Build history of the part. All positions in model axes, mm. Round coordinates to 2 decimals unless told otherwise and drop trailing zeros. Order: outer loops, then holes, each group sorted by start corner. A loop starts at its lowest first (then second) coordinate and runs counter-clockwise, first axis right, second up. Notation, with made-up numbers: (7, -30) -> (40, -30) arc R19 cw to (40, -11) -> close; hole circle Ø2 at (46.25, 24.5). An arc over 180 degrees is marked (long way). Use a Markdown table: item, result. Add a question column.
Item 1: Slice it at A-A, the plane z = 39.5. Give the cut face in (x, y).
Item 2: Pin check, flat tips, straight feed: pin 1 (2 mm diameter, centred on x = 3, z = 62, fed in from +Y); pin 2 (2.5 mm diameter, centred on y = 2, z = 70.5, fed in from -X); pin 3 (1 mm diameter, centred on x = -4, y = 4.5, fed in from +Z); pin 4 (1.6 mm diameter, centred on y = 2, z = 49.5, fed in from +X). Stop position of each tip, or through.
Item 3: Slice it at C-C, the plane z = -32. Give the cut face in (x, y), plus the area to 3 significant figures.
Item 4: Slice it at D-D, the plane y = 4.25. State how many separate pieces and enclosed holes the cut face has, plus the area to 3 significant figures.
Item 5: Probe L1, parallel to X at y = 4.55, z = 72; L2, parallel to X at y = 1.5, z = 43.5; L3, parallel to X at y = 3.25, z = 11.5. List the from-to ranges inside material, lowest first.
Item 6: Slice it at B-B, the plane x = 0. Give the cut face in (y, z), plus the area to 3 significant figures.
Autodesk Inventor part; units mm, degrees
ref_plane "YZ Plane" through (0, 0, 0) normal (1, 0, 0) x (0, 1, 0)
ref_plane "XZ Plane" through (0, 0, 0) normal (0, 1, 0) x (-1, 0, 0)
ref_plane "XY Plane" through (0, 0, 0) normal (0, 0, 1) x (1, 0, 0)
sketch "Boceto1" plane through (0, 0, 0) normal (0, 1, 0) x (-1, 0, 0)
  line L0 (26.7996, 74.6) -> (26.8, 68.8)
  line L1 (21, 68.8) -> (21, 22.2711)
  line L2 (7.5058, -28.0118) -> (9.0069, -33.6142)
  line L3 (-9.0069, -33.6142) -> (-7.5058, -28.0118)
  line L4 (-7.5058, -28.0118) -> (-9.0069, -33.6142)
  line L5 (-20.5061, -20.5061) -> (-24.6073, -24.6073)
  line L6 (-20.5061, -20.5061) -> (-24.6073, -24.6073)
  circle A0 centre (0, 0) radius 11
  line L7 (-21, 69) -> (-21, 22.2711)
  line L8 (-21, 22.2711) -> (-21, 69)
  line L9 (-26.7402, 22.2711) -> (-21, 22.2711)
  line L10 (-27, 74.8) -> (26.7996, 74.6)
  arc A1 (-9.0069, -33.6142) -> (9.0069, -33.6142) centre (0, 0) ccw
  arc A2 (-26.7402, 22.2711) -> (-24.6073, -24.6073) centre (0, 0) ccw
  arc A3 (24.6073, -24.6073) -> (26.7402, 22.2711) centre (0, 0) ccw
  line L11 (26.8, 68.8) -> (21, 68.8)
  line L12 (21, 22.2711) -> (26.7402, 22.2711)
  line L13 (-27, 74.8) -> (-27, 69)
  line L14 (-27, 69) -> (-21, 69)
  line L15 (24.6073, -24.6073) -> (20.3647, -20.3647)
  line L16 (7.5058, -28.0118) -> (7.454, -27.8187)
  line L17 (-7.5058, -28.0118) -> (-7.454, -27.8187)
  line L18 (-20.5061, -20.5061) -> (-20.3647, -20.3647)
  arc A4 (-20.3647, -20.3647) -> (-7.454, -27.8187) centre (0, 0) ccw
  arc A5 (7.454, -27.8187) -> (20.3647, -20.3647) centre (0, 0) ccw
  point P0 (0, 0)
  point P1 (0, 0)
  dimension "d3" = 53.8
  dimension "d5" = 22
  dimension "d15" = 5.8
  dimension "d16" = 46.5289
extrude "Extrusión1" add sketch "Boceto1" along normal blind 6
fillet "Empalme2" radius 1 2 edges at (27, 3, 74.8) (-26.7996, 3, 74.6)
chamfer "Chaflán1" distance 0.6 angle 45 6 edges at (27, 0, 71.3981) (26.7058, 0, 74.5047) (0.0964, 0, 74.7) (-26.5081, 0, 74.3095) (-26.7998, 0, 71.2019) (24, 0, 69)
chamfer "Chaflán2" distance 0.6 angle 45 1 edges at (21, 0, 45.6355)
chamfer "Chaflán3" distance 0.6 angle 45 1 edges at (-21, 0, 45.5355)
chamfer "Chaflán4" distance 0.6 angle 45 2 edges at (-23.6, 0, 68.8) (-23.8701, 0, 22.2711)
chamfer "Chaflán5" distance 0.6 angle 45 3 edges at (-34.7443, 0, -1.9681) (-24.1144, 0, 21.6711) (-22.486, 0, -22.486)
chamfer "Chaflán6" distance 0.6 angle 45 9 edges at (-14.4, 0, -24.9415) (-8.2563, 0, -30.813) (0, 0, -34.8) (8.2563, 0, -30.813) (14.4, 0, -24.9415) (22.5567, 0, -22.5567) (34.764, 0, -1.5817) (23.8701, 0, 22.2711) (20.4, 0, 45.6355)
fillet "Empalme4" radius 0.5 4 edges at (-9.0069, 3.2998, -33.6142) (-24.6073, 3.2998, -24.6073) (9.0069, 3.2998, -33.6142) (24.6073, 3.2998, -24.6073)
sketch "Boceto2" plane through (0, 0, 0) normal (0, -1, 0) x (1, 0, 0)
  line L0 (0, 52.5) -> (0, 37.5) construction
  line L1 (-12.5, 52.5) -> (-12.5, 37.5)
  line L2 (12.5, 37.5) -> (12.5, 52.5)
  arc A0 (12.5, 52.5) -> (-12.5, 52.5) centre (0, 52.5) ccw
  arc A1 (-12.5, 37.5) -> (12.5, 37.5) centre (0, 37.5) ccw
  point P0 (0, 0)
  point P1 (0, 45)
  dimension "d43" = 25
  dimension "d44" = 15
  dimension "d45" = 37.5
extrude "Extrusión2" cut sketch "Boceto2" against normal blind 6
sketch "Boceto3" plane through (0, 6, 0) normal (0, 1, 0) x (1, 0, 0)
  circle A0 centre (0.0066, -72) radius 1.6
  circle A1 centre (0, 0) radius 32
  circle A2 centre (0, 32) radius 1.6
  circle A3 centre (-30.0702, -10.9446) radius 1.6
  circle A4 centre (30.0702, -10.9446) radius 1.6
  line L0 (0, 0) -> (-30.0702, -10.9446)
  line L1 (0, 0) -> (30.0702, -10.9446)
  line L2 (9.4586, 0) -> (-7.7353, 0)
  dimension "d48" = 64
  dimension "d49" = 3.2
  dimension "d50" = 20
  dimension "d51" = 20
  dimension "d53" = 72
extrude "Extrusión3" cut sketch "Boceto3" against normal through all contours A0 | A2 A1 | A1 A2 | A4 A1 | A1 L1 A4 | A1 A4 L1 | A3 L0 A1 | A1 A3 | L0 A3 A1
properties part number "Tapa de caja reductora - eje z" material "Plastico PETG"
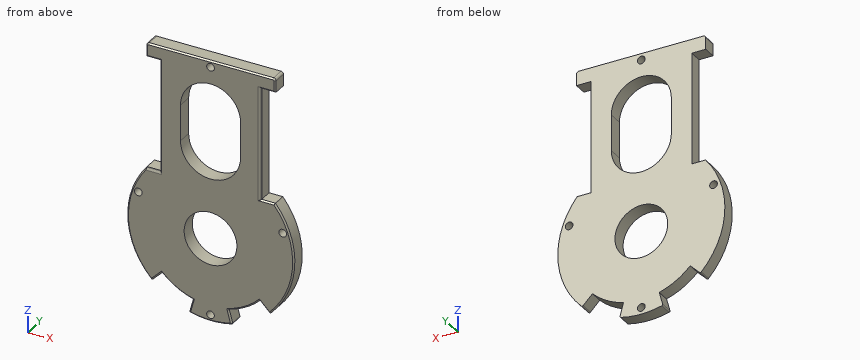
Check sheet entries:
| question | item | result |
|---|---|---|
| 1 | outline | (-21, 0.6) -> (-20.4, 0) -> (-12.5, 0) -> (-12.5, 6) -> (-21, 6) -> close; (12.5, 0) -> (19.8, 0) -> (20.82, 0.42) -> (21, 0.6) -> (21, 6) -> (12.5, 6) -> close |
| 2 | pin 1 | through |
| 2 | pin 2 | x = -26.8 |
| 2 | pin 3 | z = 74.69 |
| 2 | pin 4 | x = 21 |
| 3 | outline | (-8.57, 0.6) -> (-7.96, 0) -> (-1.6, 0) -> (-1.6, 6) -> (-8.57, 6) -> close; (1.6, 0) -> (7.96, 0) -> (8.57, 0.6) -> (8.57, 6) -> (1.6, 6) -> close |
| 3 | area | 83.3 mm2 |
| 4 | separate pieces | 1 |
| 4 | enclosed holes | 6 |
| 4 | area | 4,130 mm2 |
| 5 | L1 | -26.8 to -1.59, 1.61 to 27 |
| 5 | L2 | -21 to -12.5, 12.5 to 21 |
| 5 | L3 | -32.84 to -31.57, -28.57 to 28.57, 31.57 to 32.84 |
| 6 | outline | (0, -34.2) -> (0.6, -34.8) -> (6, -34.8) -> (6, -33.6) -> (0, -33.6) -> close; (0, -30.4) -> (6, -30.4) -> (6, -11) -> (0, -11) -> close; (0, 11) -> (6, 11) -> (6, 25) -> (0, 25) -> close; (0, 65) -> (6, 65) -> (6, 70.4) -> (0, 70.4) -> close; (0, 73.6) -> (6, 73.6) -> (6, 74.7) -> (0.6, 74.7) -> (0, 74.1) -> close |
| 6 | area | 246 mm2 |
